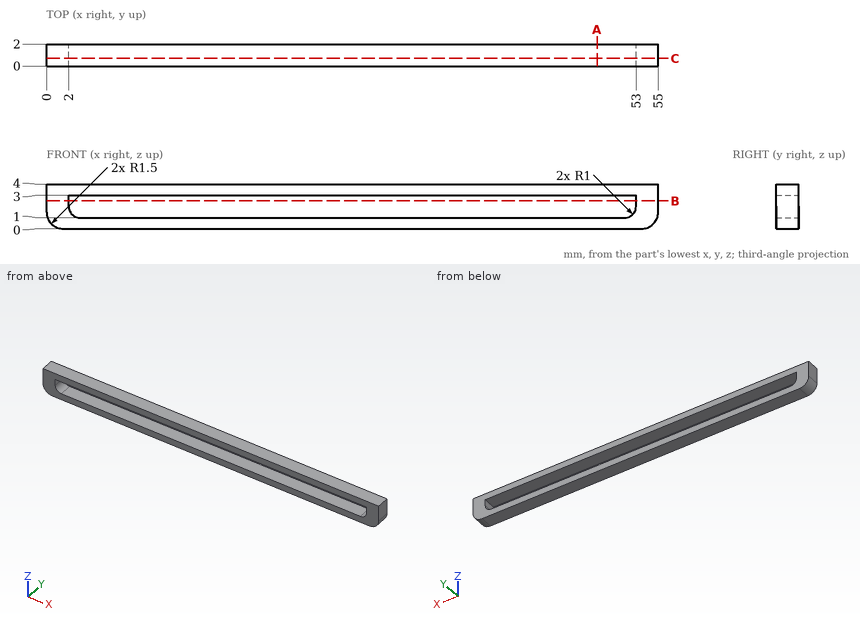
Drawing for the job (mm, zero at the part's lowest x, y, z). Give positions to 0.01 mm unless a question says otherwise; leave off trailing zeros. Write each loop counter-clockwise with the first axis right and the second up, starting at its lowest first coordinate (ties: lowest second). Pieces come first, ordered by that corner, then holes. Notation, with made-up numbers: M 2.5,89 L 36.5,89 A15 ccw 36.5,102 Z; hole C -14,-10 d6. An arc over 180 degrees is marked long. Return JSON: item names as keys, results as strings. Group by question number.
(1) Band-saw the part on B-B (z = 2.5). Give the cut face in (x, y).
(2) Drill centre lines: L1, parallel to Z at x = 16, y = 1.25; L2, parallel to X at y = 1.55, z = 2.8; L3, parallel to X at y = 0.3, z = 1.25. Where is each one in solid material? Low to high. Write a range as [from, to].
(3) Band-saw the part on A-A (x = 49.5). Give the cut face in (y, z), and give its area (3 significant figures).
(4) Band-saw the part on C-C (y = 0.7). Give the cut face in (x, z), and give its area (3 significant figures).
Entries:
{
 "1": {"outline": "M 0,0 L 2,0 L 2,2 L 0,2 Z; M 53,0 L 55,0 L 55,2 L 53,2 Z"},
 "2": {"L1": "z = [0, 1], [3, 4]", "L2": "x = [0, 2], [53, 55]", "L3": "x = [0.02, 2.34], [52.66, 54.98]"},
 "3": {"outline": "M 0,0 L 2,0 L 2,1 L 0,1 Z; M 0,3 L 2,3 L 2,4 L 0,4 Z", "area": "4.00 mm^2"},
 "4": {"outline": "M 0,1.5 A1.5 ccw 1.5,0 L 53.5,0 A1.5 ccw 55,1.5 L 55,4 L 0,4 Z; hole M 2,2 A1 ccw 3,1 L 52,1 A1 ccw 53,2 L 53,3 L 2,3 Z", "area": "117 mm^2"}
}
